The drawing under review shows one solid part. Ordinate dimensions are in mm from its lowest x, y, z. Coordinates: 2 decimals unless noted, no trailing zeros. Write each loop counter-clockwise with the first axis right and the second up, starting at its lowest first coordinate (ties: lowest second). Pieces come first, ordered by that corner, then holes.
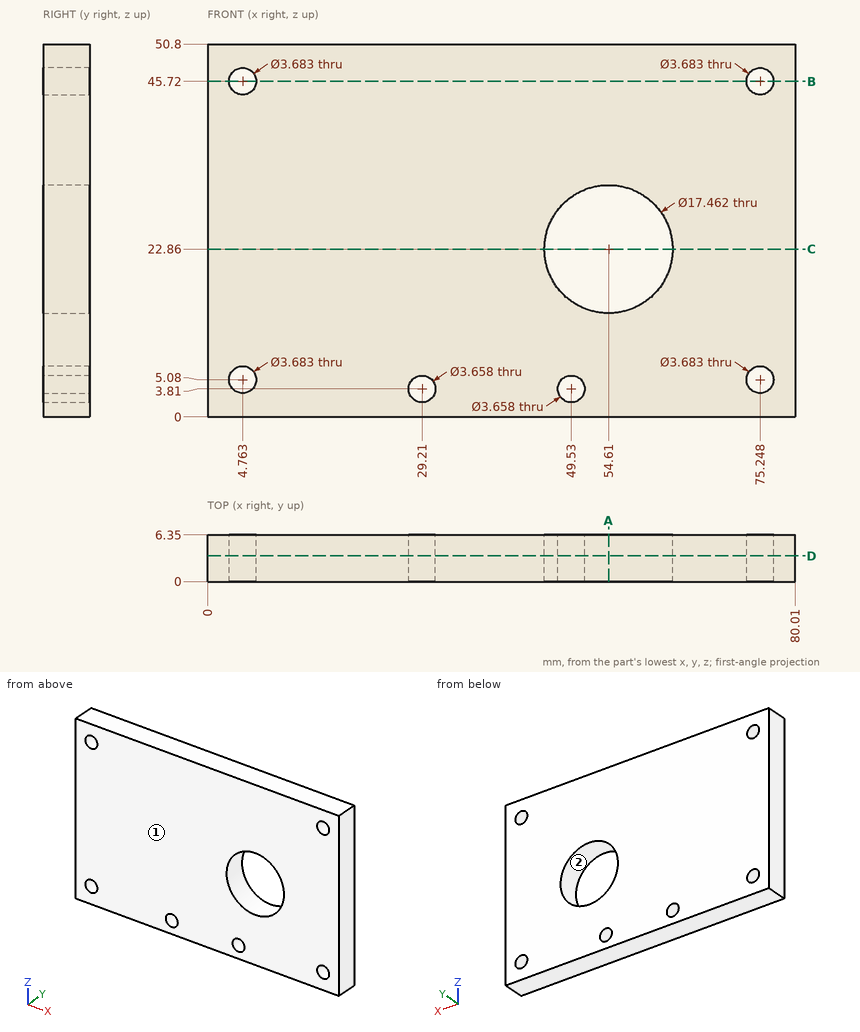
1) The part is to be moulded in two halves that separate along X. For the marked faces 1 and 2, say which applies: pulls with the +X half, pulls with the -X half, needs draft (parallel to the pull), parting line crosses it, or undercut.
2) Consider section D-D (y = 3.5). Give the boundary of the cut face in (x, z), then the cut area to 3 significant figures.
3) For L1, parallel to X at y = 2.25, z = 45.72 (1 decimal); L2, parallel to X at y = 5.25, z = 6.5 (1 decimal); L3, parallel to X at y = 2.75, z = 3.81 (1 decimal), list the stretches that pass through material, from the lowest coordinate up.
4) Consider section B-B (z = 45.72). Count the separate pieces of the cut face and the enclosed holes in it, then the cut area to 3 significant figures.
5) Consider section C-C (z = 22.86). Give the boundary of the cut face in (x, y).
6) Consider section A-A (x = 54.61). Give the boundary of the cut face in (y, z).
Results:
1. face 1: needs draft
1. face 2: undercut
2. outline: (0, 0) - (80.01, 0) - (80.01, 50.8) - (0, 50.8) - close; hole circle Ø3.68 at (4.76, 5.08); hole circle Ø3.68 at (4.76, 45.72); hole circle Ø3.66 at (29.21, 3.81); hole circle Ø17.46 at (54.61, 22.86); hole circle Ø3.66 at (49.53, 3.81); hole circle Ø3.68 at (75.25, 5.08); hole circle Ø3.68 at (75.25, 45.72)
2. area: 3,760 mm2
3. L1: x = 0 to 2.9, 6.6 to 73.4, 77.1 to 80
3. L2: x = 0 to 3.6, 5.9 to 74.1, 76.4 to 80
3. L3: x = 0 to 3.4, 6.1 to 27.4, 31 to 47.7, 51.4 to 73.9, 76.6 to 80
4. separate pieces: 3
4. enclosed holes: 0
4. area: 461 mm2
5. outline: (0, 0) - (45.88, 0) - (45.88, 6.35) - (0, 6.35) - close; (63.34, 0) - (80.01, 0) - (80.01, 6.35) - (63.34, 6.35) - close
6. outline: (0, 0) - (6.35, 0) - (6.35, 14.13) - (0, 14.13) - close; (0, 31.59) - (6.35, 31.59) - (6.35, 50.8) - (0, 50.8) - close
